Can you work these out from the model? Positions are in its coordinate system, mm. A direction names the side the tool comes from. Give positions to 0.01 mm unless a question says otherwise; leave off trailing zeros. Write each loop counter-clockwise with the first axis right and the second up, starting at its lowest first coordinate (ties: lowest second). Pieces come first, ordered by that corner, then holes. Notation, with made-up numbers: (59.25, 46) - (86.25, 46) arc R13 ccw to (86.25, 68) - close; hole circle Ø10 at (-9.5, 70). An arc over 180 degrees is marked (long way). Return JSON: item names as keys, results as strings. Group by question number.
Autodesk Inventor part; units mm, degrees
ref_plane "Work Plane1" through (29, 0, 0) normal (0, -1, 0) x (1, 0, 0)
ref_plane "YZ Plane" through (0, 0, 0) normal (1, 0, 0) x (0, 1, 0)
ref_plane "XZ Plane" through (0, 0, 0) normal (0, 1, 0) x (-1, 0, 0)
sketch "Sketch1" plane through (0, 0, 0) normal (0, 0, 1) x (1, 0, 0)
  line L0 (-1, 0) -> (50, 0)
  line L1 (50, 0) -> (50, 2)
  line L2 (50, 2) -> (30, 2)
  line L3 (30, 2) -> (29.5705, 2)
  line L4 (29.5705, 2) -> (0, 2)
  line L5 (0, 2) -> (0, 3.5)
  line L6 (0, 3.5) -> (-4, 3.5)
  line L7 (-4, 3.5) -> (-4, 1.7321)
  line L8 (-4, 1.7321) -> (-2, 1.7321)
  line L9 (-2, 1.7321) -> (-1, 0)
  line L10 (-14.8, 0) -> (60.8, 0)
  line L11 (0, -0.7) -> (0, 4.2)
  line L12 (30, 2) -> (0, 2) construction
  dimension "d1" = 20
  dimension "d2" = 0.4295
  dimension "d3" = 4
  dimension "d4" = 2
  dimension "d5" = 60
  dimension "d6" = 4
  dimension "d7" = 4
  dimension "d8" = 3.4641
  dimension "d9" = 7
  dimension "d26" = 50
revolve "Body" add sketch "Sketch1" angle 360 about axis through (-1, 0, 0) along (1, 0, 0)
sketch "Sketch2" plane through (-4, 0, 0) normal (-1, 0, 0) x (0, 0, 1)
  circle A0 centre (0, 0) radius 1.7321
  line L0 (0, -4.9) -> (0, 4.9)
  line L1 (-4.9, 0) -> (4.9, 0)
  line L2 (1.7321, 0) -> (0.866, -1.5)
  line L3 (0.866, -1.5) -> (-0.866, -1.5)
  line L4 (-0.866, -1.5) -> (-1.7321, 0)
  line L5 (-1.7321, 0) -> (-0.866, 1.5)
  line L6 (-0.866, 1.5) -> (0.866, 1.5)
  line L7 (0.866, 1.5) -> (1.7321, 0)
extrude "Slot" add sketch "Sketch2" against normal up to next contours L7 A0 | A0 L2 | L6 L0 A0 | A0 L0 L3 | L0 L6 A0 | A0 L3 L0 | L4 A0 | A0 L5
fillet "Fillet1" radius 0.35 1 edges at (-4, -3.5, 0)
thread "Thread"
chamfer "Chamfer1" distance 0.4294 distance2 0.4294 1 edges at (50, -2, 0) measured on face at (50, -0.8158, 0.4805)
ref_plane "Work Plane1" through (29, 0, 0) normal (0, -1, 0) x (1, 0, 0)
fillet "Fillet2" radius 0.1 1 edges at (0, -2, 0)
equation "\"d1\" = GEL"
equation "\"d3\" = KOH"
equation "\"d4\" = INTI"
equation "\"d6\" = GD"
equation "\"d7\" = BDM"
equation "\"d8\" = 1.1547 * SW"
equation "\"d9\" = KOD"
equation "\"d26\" = NLG"
equation "\"d30\" = R"
equation "\"d17\" = RR"
equation "\"d13\" = GEL"
equation "\"d15\" = -0.5 * SPD + 0.5 * GD"
equation "\"d16\" = GUL"
equation "\"GD\" = NND"
equation "\"NLG\" = 50"
equation "\"GEL\" = 20"
equation "\"KOD\" = 7"
equation "\"KOH\" = NND"
equation "\"INTI\" = 2"
equation "\"GAL\" = 0.61345 * PTC"
equation "\"GUL\" = 0.61345 * PTC"
equation "\"BDM\" = NND"
equation "\"SW\" = 3"
equation "\"RR\" = 0.35"
equation "\"SPD\" = NND - 1.2269 * PTC"
equation "\"R\" = 0.1"
equation "\"PHH\" = 0.1 * NND"
equation "\"GD1\" = THREADDIA - 1.2269 * PTC"
equation "\"THREADDIA\" = 4"
equation "\"FAWI\" = 45deg"
equation "\"PTC\" = 0.7"
equation "\"NND\" = 4"
equation "\"FAWI1\" = 30deg"
equation "\"TOA\" = 30deg"
equation "\"E0\" = 1.155 * SW"
properties part number "Unbrako - M4 x 50" material "Steel, Mild"
1) We'd pull the mould along Z, two halves only. Please class faces 1 (the face through (-2.948, -0.74, 1.305)), 2 (the face through (-1.851, 3.233, 1.341)), 3 (the face through (50, 0, 0)): pulls with the +Z half, pulls with the -Z half, needs draft (parallel to the pull), parting line crosses it, or undercut.
2) On a 3-axis mill with a long thin cutter (end or side, diameter ignored), from which of +Z, -Z, +X, -X, +Y, -Y can I reach the whole of each face in a straight line? I mean faces 4 (the face through (-4, -1.4, 1.4)), 5 (the face through (-2.948, 0.761, 1.293)), 6 (the face through (24, 0, 2)). Say none if no direction works.
3) Imagine slicing it at A-A, the plane x = 44. Write out the boundary of the cut face in (y, z), and give its area (3 significant figures).
4) Will these pins go through, and if not, where does the flat tip stop? pin 1 Ø2 at (x, y) = (25, 0.5) entering from -Z; pin 2 Ø3 at (x, z) = (35.5, -0.5) entering from +Y.
5) I need wall thicknesses on line 1 along Y through (x, z) = (1, -1); line 2 along Y through (x, z) = (4, 1.25); line 3 along X through (y, z) = (-1, 0). Which ranges of each line are inside material? Lowest first, please.
Resolved:
{
 "1": {"face 1": "undercut", "face 2": "parting line crosses it", "face 3": "needs draft"},
 "2": {"face 4": "+Z, -Z, -X, +Y, -Y", "face 5": "-X", "face 6": "+X"},
 "3": {"outline": "circle Ø4 at (0, 0)", "area": "12.6 mm^2"},
 "4": {"pin 1": "z = -2", "pin 2": "y = 2"},
 "5": {"line 1": "-1.73 to 1.73", "line 2": "-1.56 to 1.56", "line 3": "-1.58 to 50"}
}
